Read the model definition and answer for the solid it produces. Units are mm, in the model's axes. A direction names the side the tool comes from. Coordinates: 2 decimals unless noted, no trailing zeros. Order: outer loops, then holes, each group sorted by start corner. A loop starts at its lowest first (then second) coordinate and runs counter-clockwise, first axis right, second up. Notation, with made-up numbers: M -27.5,3.25 L -9.5,3.25 A33 cw -9.5,37.25 Z; hole C 23,52 d7. An arc over 180 degrees is marked long. One line per question, with ' | ' between items. Start each with the question number.
1) Find section A-A, the plane x = -79. Write down the section's boundary in (y, z).
2) Consider probe 1 along Y at (x, z) = (65.5, 14); probe 2 along X at (y, z) = (-1, 88); probe 3 along X at (y, z) = (0, 77). Determine where each line is inside the solid, lowest interval first.
3) Given P1, Ø3, axis at x = -244, y = -19, coming from the +Z side; P2, Ø12, axis at y = 11.5, z = 65, coming from the +X side; P3, Ø4, axis at y = 14, z = 61, coming from the -X side; P4, Ø12, axis at y = 2, z = 66.5, coming from the +X side, each flat-ended and moving along its own axis, determine where each tip first touches the part or whether it passes through.
4) Find section B-B, the plane z = 34. Write down the section's boundary in (x, y), plus the area to 3 significant figures.
5) Find section C-C, the plane y = -12. Write down the section's boundary in (x, z).
6) The mould has two halves that part along X. Classify faces 3 (the face through (98.65, -1.56, 49.3)), 4 (the face through (-145, 19, 0)), 5 (the face through (-393.34, -2.48, 49.3)), 6 (the face through (100.648, -1.516, 49.3)): +X half, -X half, draft (parallel to the pull), parting line (faces both ways), or undercut.
7) A tool of negligible diameter and unlimited length cuts with its end or side. For faces 1 (the face through (-143, -24, 49)), 2 (the face through (-149, 18, 49)), from which of +Z, -Z, +X, -X, +Y, -Y can it reach the whole face along a straight path? Write none if from no direction.
from build123d import *

# Parameters (mm, degrees)
BOSS_EXTRUDE1_DEPTH = 100
SHELL2_T            = -2


with BuildPart() as part:
    # Sketch1 → Boss-Extrude1 (new body)
    with BuildSketch(Plane.XY):
        with BuildLine():
            Line((-371.346770179, 20), (78.653229821, 20))
            ThreePointArc((78.653229821, 20), (100.653229821, -2), (78.653229821, -24))
            Line((78.653229821, -24), (-371.346770179, -24))
            ThreePointArc((-371.346770179, -24), (-393.346770179, -2), (-371.346770179, 20))
        make_face()
    extrude(amount=BOSS_EXTRUDE1_DEPTH)

    # Shell2
    shell2_openings = [part.faces().sort_by_distance(p)[0] for p in [
        (-146.346770179, -2, 100),
        (-146.346770179, -2, 0),
    ]]
    offset(amount=SHELL2_T, openings=shell2_openings, kind=Kind.INTERSECTION)


solid = part.part
Report:
1) outline: M -24,0 L -22,0 L -22,100 L -24,100 Z; M 18,0 L 20,0 L 20,100 L 18,100 Z
2) probe 1: y = -24 to -22, 18 to 20 | probe 2: x = -393.32 to -391.32, 98.63 to 100.63 | probe 3: x = -393.26 to -391.25, 98.55 to 100.56
3) P1: passes through | P2: stops at x = 99.34 | P3: stops at x = -388.32 | P4: stops at x = 100.65
4) outline: M -371.35,-24 L 78.65,-24 A22 ccw 78.65,20 L -371.35,20 A22 ccw Z; hole M -371.35,-22 L 78.65,-22 A20 ccw 78.65,18 L -371.35,18 A20 ccw Z | area: 2,060 mm^2
5) outline: M -390.94,0 L -388.67,0 L -388.67,100 L -390.94,100 Z; M 95.97,0 L 98.25,0 L 98.25,100 L 95.97,100 Z
6) face 3: undercut | face 4: draft | face 5: -X half | face 6: +X half
7) face 1: +Z, -Z, +X, -X, -Y | face 2: +Z, -Z
